```python
from build123d import *

# Parameters (mm, degrees)
F0_W     = 38.1
F0_H     = 6.35
F0_R     = 1.905
F1_DEPTH = 6.35
F2_R     = 1.905
F3_DEPTH = 6.35


# Not quite as in the source:
# - a feature names something its author has since deleted; it is built from what else it names


with BuildPart() as f1:
    # F0 (on Front) → F1 (new body)
    with BuildSketch(Plane.XZ):
        with Locations((-18.2288356441, -3.7045082716)):
            Rectangle(F0_W, F0_H)
        with Locations((-2.3538356441, -3.7045082716)):
            Circle(F0_R, mode=Mode.SUBTRACT)
    extrude(amount=F1_DEPTH)

    # F2 (on face) → F3 (cut)
    with BuildSketch(Plane.XY.offset(-0.5295082716)):
        with Locations((-34.1285004571, -3.175)):
            Circle(F2_R)
    extrude(amount=-F3_DEPTH, mode=Mode.SUBTRACT)


solid = f1.part
```
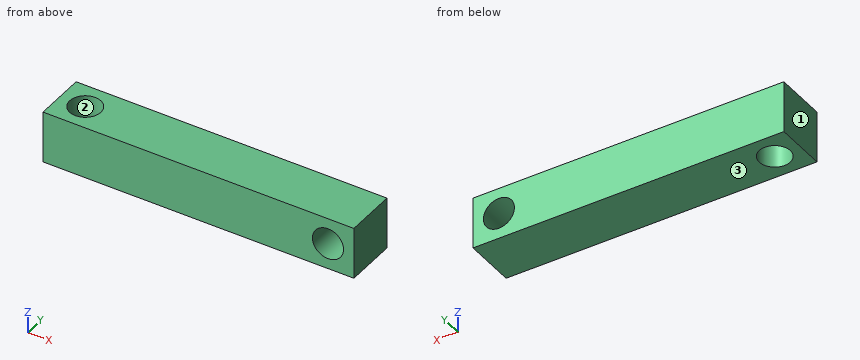
Verification items for the finished model (mm, model axes). Face numbers are marked on the shaded views. Give positions to 0.01 mm unless a question says otherwise; leave off trailing zeros. Order: outer loops, then holes, each group sorted by start corner. A loop starts at its lowest first (then second) coordinate and runs counter-clockwise, first axis right, second up. Notation, with made-up numbers: M 75.25,8.5 L 93.25,8.5 A9 cw 93.25,16.5 Z; hole C 41,41.25 d6. An arc over 180 degrees is marked long. Answer in a Markdown table with one row per item. Add a question column.
Item 1: Section check A-A, the plane z = -3. State how many separate pieces and enclosed holes the cut face has, and give its area (3 significant figures).
Item 2: Scan lines: probe 1 along X at (y, z) = (-2, -3.25); probe 2 along X at (y, z) = (-2.5, -5); probe 3 along X at (y, z) = (-3.25, -0.75). Record each from-to range of solid material in increasing order. Write a range as from..to.
Item 3: Section check B-B, the plane y = -4.75. Enter the section's corners in (x, z) (1 decimal).
Item 4: Mould release check, pull along X, two halves, no side actions. Record for the marked faces 1, 2 and 3: released by +X, released by -X, zero draft, split by the parting line, or undercut.
Filled sheet:
| question | item | result |
|---|---|---|
| 1 | separate pieces | 2 |
| 1 | enclosed holes | 1 |
| 1 | area | 208 mm^2 |
| 2 | probe 1 | x = -37.28..-35.63, -32.63..-4.2, -0.5..0.82 |
| 2 | probe 2 | x = -37.28..-35.91, -32.35..-3.75, -0.96..0.82 |
| 2 | probe 3 | x = -37.28..-36.03, -32.22..0.82 |
| 3 | outline | M -37.3,-6.9 L -35.2,-6.9 L -35.2,-0.5 L -37.3,-0.5 Z; M -33.1,-6.9 L 0.8,-6.9 L 0.8,-0.5 L -33.1,-0.5 Z; hole C -2.4,-3.7 d3.8 |
| 4 | face 1 | released by -X |
| 4 | face 2 | undercut |
| 4 | face 3 | zero draft |
